Verification items for this drawing (mm, ordinates from the low corner). A direction names the side the tool comes from. Coordinates: 2 decimals unless noted, no trailing zeros. Write each loop counter-clockwise with the first axis right and the second up, starting at its lowest first coordinate (ties: lowest second). Pieces come first, ordered by that corner, then holes. Notation, with made-up numbers: M -2,3 L 39,3 A29 cw 39,39 Z; hole C 21.25,48.25 d2. An arc over 180 degrees is marked long. Answer as CSV lines item,"result". Start each with the question number.
1) Section check B-B (z = 58). Record the cut outline in (x, y), and give its area (3 significant figures).
2) Section check C-C (y = 73.5). Record the cut outline in (x, z), and give its area (3 significant figures).
3) Section check A-A (x = 53). Record the cut outline in (y, z).
4) Material ranges on L1, parallel to Z at x = 85.5, y = 45; L2, parallel to X at y = 122.5, z = 119.5, recorded low to high. Write a range as [from, to].
5) Go/stop test with a flat-tipped pin: pin 1 Ø3 at (x, z) = (90, 101.5) entering from -Y. Record where the tip stops, or that it passes through.
6) Access from +Z, -Z, +X, -X, +Y, -Y to the whole of each face (thin tool, end or side, straight path). Record for the marked faces 1 and 2.
7) Draft check along X on the marked faces 3, 4, 5 and 6. Enter one of: +X half, -X half, draft (parallel to the pull), parting line (faces both ways), or undercut.
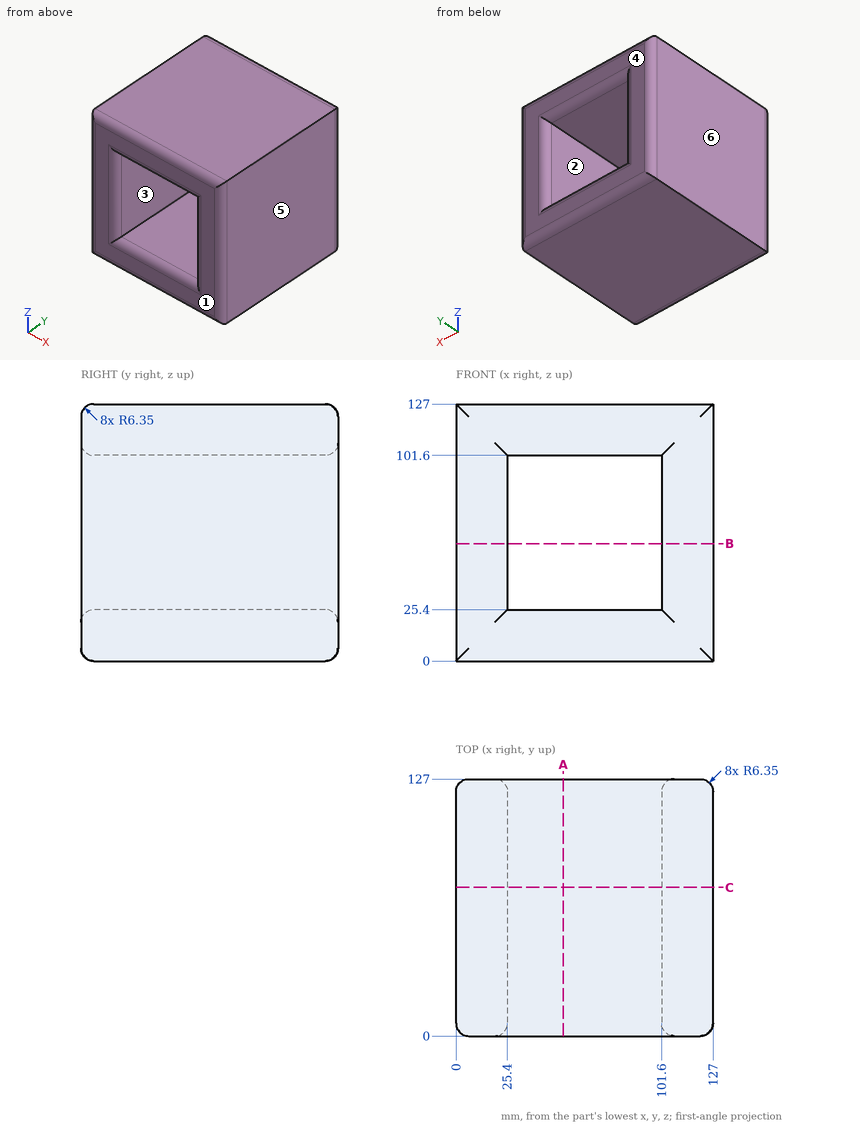
Results found:
1,outline,"M 0,6.35 A6.35 ccw 6.35,0 L 19.05,0 A6.35 ccw 25.4,6.35 L 25.4,120.65 A6.35 ccw 19.05,127 L 6.35,127 A6.35 ccw 0,120.65 Z; M 101.6,6.35 A6.35 ccw 107.95,0 L 120.65,0 A6.35 ccw 127,6.35 L 127,120.65 A6.35 ccw 120.65,127 L 107.95,127 A6.35 ccw 101.6,120.65 Z"
1,area,"6,380 mm2"
2,outline,"M 0,0 L 127,0 L 127,127 L 0,127 Z; hole M 25.4,25.4 L 101.6,25.4 L 101.6,101.6 L 25.4,101.6 Z"
2,area,"10,300 mm2"
3,outline,"M 0,6.35 A6.35 ccw 6.35,0 L 120.65,0 A6.35 ccw 127,6.35 L 127,19.05 A6.35 ccw 120.65,25.4 L 6.35,25.4 A6.35 ccw 0,19.05 Z; M 0,107.95 A6.35 ccw 6.35,101.6 L 120.65,101.6 A6.35 ccw 127,107.95 L 127,120.65 A6.35 ccw 120.65,127 L 6.35,127 A6.35 ccw 0,120.65 Z"
4,L1,"z = [0, 25.4], [101.6, 127]"
4,L2,"x = [0.28, 126.72]"
5,pin 1,"stops at y = 2.37"
6,face 1,"+Z, -Z, +X, -X, -Y"
6,face 2,"+Y, -Y"
7,face 3,"undercut"
7,face 4,"draft"
7,face 5,"+X half"
7,face 6,"-X half"
